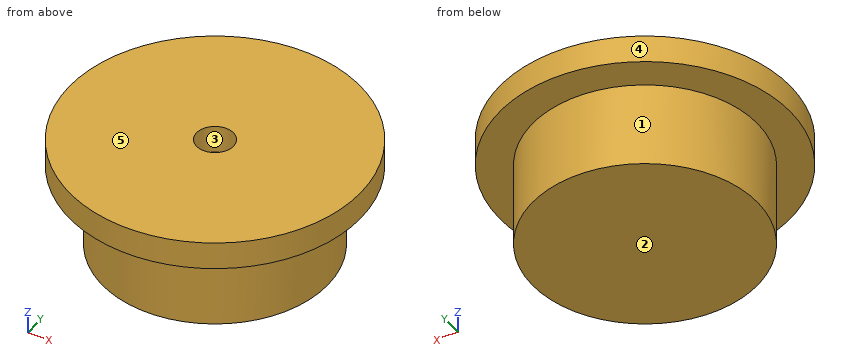
from build123d import *

# Parameters (mm, degrees)
SKETCH128_R   = 71
SKETCH128_R_2 = 9
PAD050_DEPTH  = 13.5
SKETCH131_R   = 55
PAD052_DEPTH  = 55


with BuildPart() as part:
    # Sketch128 → Pad050 (new body)
    with BuildSketch(Plane.XY):
        Circle(SKETCH128_R)
        Circle(SKETCH128_R_2, mode=Mode.SUBTRACT)
    extrude(amount=-PAD050_DEPTH)

    # Sketch131 → Pad052 (join)
    with BuildSketch(Plane.XY):
        Circle(SKETCH131_R)
    extrude(amount=-PAD052_DEPTH)

    # Sketch130 → Groove (revolve, cut)
    with BuildSketch(Plane.XZ):
        Polygon((0, 0), (9, 0), (9, -13.5), (4, -13.5), (4, -35.5), (0, -35.5), align=None)
    revolve(axis=Axis((0, 0, 0), (0, 0, 1)), mode=Mode.SUBTRACT)


solid = part.part
Part model, mm, in its own coordinate system. Face numbers are marked on the shaded views. A direction names the side the tool comes from. Give positions to 0.01 mm unless a question says otherwise; leave off trailing zeros. Order: outer loops, then holes, each group sorted by start corner. A loop starts at its lowest first (then second) coordinate and runs counter-clockwise, first axis right, second up. Notation, with made-up numbers: (6, -21.5) -> (37, -21.5) arc R25 cw to (37, 7.5) -> close; hole circle Ø1 at (20.25, -1.75). An arc over 180 degrees is marked (long way). Use one line per item in the form item = value.
(1) Pull direction X, two halves, no side cores. Call the marked faces 3, 4 and 5: +X half, -X half, draft (parallel to the pull), parting line (faces both ways), or undercut.
Solution:
face_3 = undercut
face_4 = parting line
face_5 = draft
(2) Tool access for the marked faces 1 and 2: list every direction of +Z, -Z, +X, -X, +Y, -Y with a clear straight run to the whole face (end or side of a thin tool).
Solution:
face_1 = -Z
face_2 = -Z, +X, -X, +Y, -Y
(3) Flat gauge pins, fed straight in: P1, Ø2, axis at y = -38.5, z = -20.5, coming from the -X side; P2, Ø9, axis at x = 0.5, y = 2, coming from the +Z side; P3, Ø1, axis at x = -41, y = -48.5, coming from the -Z side. Where does each tip first touch, or does it go through?
Solution:
P1 = -40.23
P2 = -13.5
P3 = -13.5
(4) Drill centre lines: line 1 (Y direction, x = 0, z = -26.5); line 2 (Z direction, x = 35, y = -60.5); line 3 (X direction, y = 44.5, z = -50). Where is each one in solid material? Low to high. Write a range as from..to.
Solution:
line_1 = -55..-4, 4..55
line_2 = -13.5..0
line_3 = -32.32..32.32
(5) Saw through at D-D (y = 26). Write the cut outline in (x, z).
Solution:
outline = (-66.07, -13.5) -> (-48.47, -13.5) -> (-48.47, -55) -> (48.47, -55) -> (48.47, -13.5) -> (66.07, -13.5) -> (66.07, 0) -> (-66.07, 0) -> close
(6) Saw through at A-A (x = 0). Write the cut outline in (y, z).
Solution:
outline = (-71, -13.5) -> (-55, -13.5) -> (-55, -55) -> (55, -55) -> (55, -13.5) -> (71, -13.5) -> (71, 0) -> (9, 0) -> (9, -13.5) -> (4, -13.5) -> (4, -35.5) -> (-4, -35.5) -> (-4, -13.5) -> (-9, -13.5) -> (-9, 0) -> (-71, 0) -> close
(7) Saw through at C-C (z = -6.5). Write the cut outline in (x, y), then the cut area to 3 significant figures.
Solution:
outline = circle Ø142 at (0, 0); hole circle Ø18 at (0, 0)
area = 15,600 mm²
